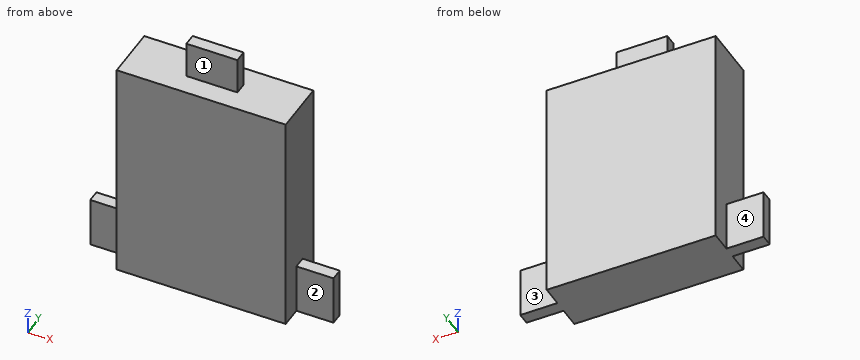
```python
from build123d import *

# Parameters (mm, degrees)
SKETCH1_W           = 25.01
SKETCH1_H           = 33.905
BOSS_EXTRUDE1_DEPTH = 8
SKETCH2_W           = 7.55
SKETCH2_H           = 1.8
BOSS_EXTRUDE2_DEPTH = 5.495
SKETCH3_W           = 7.55
SKETCH3_H           = 1.8
BOSS_EXTRUDE3_DEPTH = 5.495


with BuildPart() as part:
    # Sketch1 → Boss-Extrude1 (new body)
    with BuildSketch(Plane(origin=(0, 0, 0), x_dir=(1, 0, 0), z_dir=(0, 1, 0))):
        Rectangle(SKETCH1_W, SKETCH1_H)
    extrude(amount=BOSS_EXTRUDE1_DEPTH)

    # Sketch2 → Boss-Extrude2 (add)
    with BuildSketch(Plane.XY.offset(16.9525)):
        with Locations((0, 4)):
            Rectangle(SKETCH2_W, SKETCH2_H)
    extrude(amount=BOSS_EXTRUDE2_DEPTH)

    # Sketch3 → Boss-Extrude3 (add)
    with BuildSketch(Plane.ZY.offset(12.505)):
        with Locations((-13.1775, 4)):
            Rectangle(SKETCH3_W, SKETCH3_H)
    boss_extrude3 = extrude(amount=BOSS_EXTRUDE3_DEPTH)

    # Mirror2: Boss-Extrude3 across plane
    add(boss_extrude3.mirror(Plane(origin=(0, 0, 0), x_dir=(0, 0, 1), z_dir=(1, 0, 0))))


solid = part.part
```
Model file for the job. Use its own axes, mm. Face numbers are marked on the shaded views. A direction names the side the tool comes from. Coordinates: 2 decimals unless noted, no trailing zeros. Loops run counter-clockwise (first coordinate to the right, second up) from the corner with the lowest first, then second, coordinate; pieces in that order, holes last. Notation, with made-up numbers: M 38,58.5 L 66,58.5 A22 cw 66,82.5 Z; hole C 50,-5.75 d3. An arc over 180 degrees is marked long. Use CSV: the item, a comma, the result in double quotes. Start each with the question number.
1. Band-saw the part on D-D, the plane x = 5. List the corners of the cut face in (y, z), then the cut area to 3 significant figures.
2. Band-saw the part on A-A, the plane x = 0. List the corners of the cut face in (y, z).
3. Tool access for the marked faces 1, 2, 3 and 4: list every direction of +Z, -Z, +X, -X, +Y, -Y with a clear straight run to the whole face (end or side of a thin tool).
4. Probe probe 1 along Z at (x, y) = (4.5, 7); probe 2 along X at (y, z) = (3.5, 6.5) (3 decimals); probe 3 along Y at (x, z) = (15, -13.5). List the from-to ranges inside material, lowest first. Write a range as [from, to].
5. Flat gauge pins, fed straight in: pin 1 (0.9 mm diameter, centred on y = 4, z = 19.5, fed in from -X) (3 decimals); pin 2 (2 mm diameter, centred on y = 4.5, z = 3.5, fed in from -X) (3 decimals); pin 3 (1.4 mm diameter, centred on x = -14.5, y = 4.5, fed in from +Z). Where does each tip first touch, or does it go through?
6. Band-saw the part on B-B, the plane z = -13. List the corners of the cut face in (x, y) (3 decimals), then the cut area to 3 significant figures.
7. Band-saw the part on C-C, the plane y = 4. List the corners of the cut face in (x, z) (1 decimal), then the cut area to 3 significant figures.
Entries:
1,outline,"M 0,-16.95 L 8,-16.95 L 8,16.95 L 0,16.95 Z"
1,area,"271 mm2"
2,outline,"M 0,-16.95 L 8,-16.95 L 8,16.95 L 4.9,16.95 L 4.9,22.45 L 3.1,22.45 L 3.1,16.95 L 0,16.95 Z"
3,face 1,"+Z, +X, -X, -Y"
3,face 2,"+Z, -Z, +X, -Y"
3,face 3,"+Z, -Z, +X, +Y"
3,face 4,"+Z, -Z, -X, +Y"
4,probe 1,"z = [-16.95, 16.95]"
4,probe 2,"x = [-12.505, 12.505]"
4,probe 3,"y = [3.1, 4.9]"
5,pin 1,"stops at x = -3.775"
5,pin 2,"stops at x = -12.505"
5,pin 3,"stops at z = -9.4"
6,outline,"M -18,3.1 L -12.505,3.1 L -12.505,0 L 12.505,0 L 12.505,3.1 L 18,3.1 L 18,4.9 L 12.505,4.9 L 12.505,8 L -12.505,8 L -12.505,4.9 L -18,4.9 Z"
6,area,"220 mm2"
7,outline,"M -18,-17 L 18,-17 L 18,-9.4 L 12.5,-9.4 L 12.5,17 L 3.8,17 L 3.8,22.4 L -3.8,22.4 L -3.8,17 L -12.5,17 L -12.5,-9.4 L -18,-9.4 Z"
7,area,"972 mm2"
